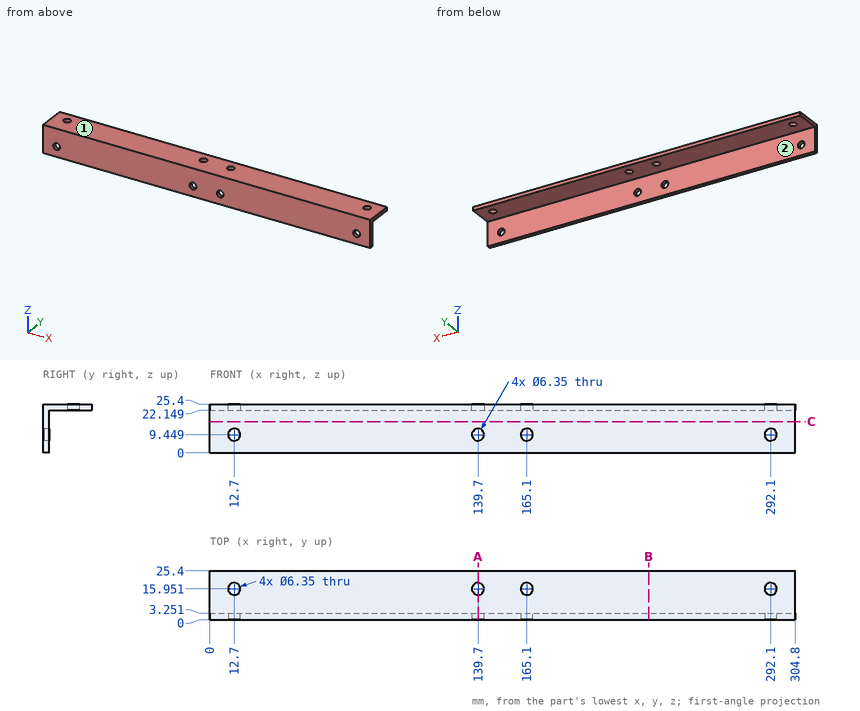
Job drawing, mm, ordinate dimensions from the low corner. One solid piece. A direction names the side the tool comes from. Give positions to 0.01 mm unless a question says otherwise; leave off trailing zeros. Order: outer loops, then holes, each group sorted by start corner. A loop starts at its lowest first (then second) coordinate and runs counter-clockwise, first axis right, second up. Notation, with made-up numbers: (23.5, 84) - (63.5, 84) arc R12 cw to (63.5, 90) - close; hole circle Ø6 at (-2, -19). An arc over 180 degrees is marked (long way). One line per question, with ' | ' between items.
1. Band-saw the part on B-B on x = 228.5. List the corners of the cut face in (y, z), then the cut area to 3 significant figures.
Filled in:
outline: (0, 0) - (3.25, 0) - (3.25, 22.15) - (25.4, 22.15) - (25.4, 25.4) - (0, 25.4) - close | area: 155 mm²
2. Band-saw the part on C-C on z = 16.25. List the corners of the cut face in (x, y).
Filled in:
outline: (0, 0) - (304.8, 0) - (304.8, 3.25) - (0, 3.25) - close
3. Band-saw the part on A-A on x = 139.7. List the corners of the cut face in (y, z).
Filled in:
outline: (0, 0) - (3.25, 0) - (3.25, 6.27) - (0, 6.27) - close; (0, 12.62) - (3.25, 12.62) - (3.25, 22.15) - (12.78, 22.15) - (12.78, 25.4) - (0, 25.4) - close; (19.13, 22.15) - (25.4, 22.15) - (25.4, 25.4) - (19.13, 25.4) - close
4. Drill centre lines: probe 1 along Z at (x, y) = (165.1, 2.3); probe 2 along Y at (x, z) = (139.7, 24.25); probe 3 along Z at (x, y) = (146.5, 15). Where is each one in solid material? Low to high.
Filled in:
probe 1: 0 to 6.27, 12.62 to 25.4 | probe 2: 0 to 12.78, 19.13 to 25.4 | probe 3: 22.15 to 25.4
5. Which spindle directions (+Z, -Z, +X, -X, +Y, -Y) get a long thin tool onto all of the face, cutting with end or side? Do the marked faces 1 and 2. Say none if no direction does.
Filled in:
face 1: +Z, +X, -X, +Y, -Y | face 2: -Z, +X, -X, +Y
6. Drop flat-ended pins along their axis: P1, Ø6.5, axis at x = 212.5, z = 12, coming from the +Y side; P2, Ø1.5, axis at x = 106.5, y = 20, coming from the -Z side. Give the stop position or say it passes through.
Filled in:
P1: y = 3.25 | P2: z = 22.15
